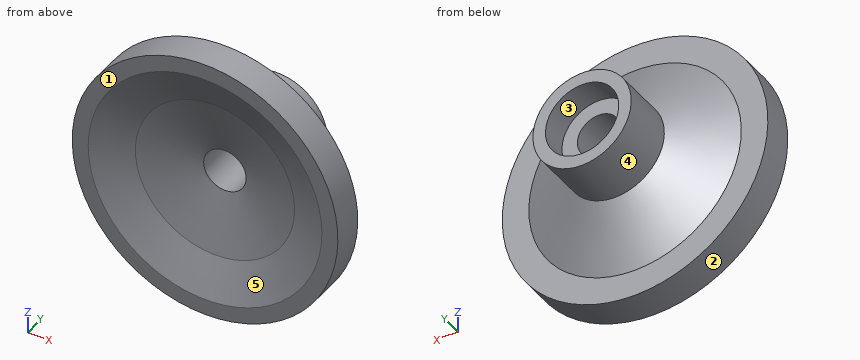
from build123d import *

# Parameters (mm, degrees)
SKETCH5_R          = 22
SKETCH7_R          = 15
SKETCH10_R         = 4
CUT_EXTRUDE1_DEPTH = 20
SKETCH11_R         = 6.9
CUT_EXTRUDE2_DEPTH = 5


with BuildPart() as part:
    # Sketch4 → Revolve1 (revolve)
    with BuildSketch(Plane.XY, mode=Mode.PRIVATE) as revolve1_sk:
        Polygon((25, 0), (25, 6), (20, 6), (9.25, 12), (9.25, 22), (0, 22), (0, 0), align=None)
    revolve(revolve1_sk.sketch.rotate(Axis((0, 0, 0), (0, 1, 0)), 90), axis=Axis((0, 0, 0), (0, 1, 0)))

    # Sketch5 → Cut-Loft1 section 0
    with BuildSketch(Plane.XZ):
        Circle(SKETCH5_R)
    # Sketch7 → Cut-Loft1 section 1
    with BuildSketch(Plane(origin=(0, 3, 0), x_dir=(-1, 0, 0), z_dir=(0, -1, 0))):
        Circle(SKETCH7_R)
    loft(mode=Mode.SUBTRACT)

    # Cut-Loft2: read off the stored shape, not the designer's step
    # Cut-Loft2: loft between two sections, ruled curve by curve
    cut_loft2_from = [
        Edge.make_bspline([(-3.999744183, 6, 0.04523797), (-4.090220122, 6, -7.954250395), (3.909268243, 6, -8.044726335), (3.999744183, 6, -0.04523797), (4.090220122, 6, 7.954250395), (-3.909268243, 6, 8.044726335), (-3.999744183, 6, 0.04523797)], [0, 0, 0, 0, 0.5, 0.5, 0.5, 1, 1, 1, 1], 3, [1, 0.333333333, 0.333333333, 1, 0.333333333, 0.333333333, 1]),
    ]
    cut_loft2_to = [
        Edge.make_bspline([(-14.242368289, 3, 4.706904028), (-23.656176345, 3, -23.777832549), (4.828560232, 3, -33.191640605), (14.242368289, 3, -4.706904028), (23.656176345, 3, 23.777832549), (-4.828560232, 3, 33.191640605), (-14.242368289, 3, 4.706904028)], [0, 0, 0, 0, 0.5, 0.5, 0.5, 1, 1, 1, 1], 3, [1, 0.333333333, 0.333333333, 1, 0.333333333, 0.333333333, 1]),
    ]
    cut_loft2 = Solid(Shell([*[Face.make_surface_from_curves(cut_loft2_from[k], cut_loft2_to[k]) for k in range(1)], Face(Wire(cut_loft2_from)), Face(Wire(cut_loft2_to))]))
    add(cut_loft2, mode=Mode.SUBTRACT)

    # Sketch10 → Cut-Extrude1 (cut)
    with BuildSketch(Plane.XZ.offset(-6)):
        with Locations(Location((0, 0, 0), (0, 0, 179.352))):
            Circle(SKETCH10_R)
    extrude(amount=-CUT_EXTRUDE1_DEPTH, mode=Mode.SUBTRACT)

    # Sketch11 → Cut-Extrude2 (cut)
    with BuildSketch(Plane(origin=(0, 22, 0), x_dir=(1, 0, 0), z_dir=(0, 1, 0))):
        with Locations(Location((0, 0, 0), (0, 0, 270))):
            Circle(SKETCH11_R)
    extrude(amount=-CUT_EXTRUDE2_DEPTH, mode=Mode.SUBTRACT)


solid = part.part
Here's how the part is built. I have some questions about the finished solid (model axes, mm). Face numbers are marked on the shaded views. A direction names the side the tool comes from. Coordinates: 2 decimals unless noted, no trailing zeros. Write each loop counter-clockwise with the first axis right and the second up, starting at its lowest first coordinate (ties: lowest second). Pieces come first, ordered by that corner, then holes.
Item 1: On a 3-axis mill with a long thin cutter (end or side, diameter ignored), from which of +Z, -Z, +X, -X, +Y, -Y can I reach the whole of each face in a straight line? I mean the marked faces 4 and 5. Say none if no direction works.
Item 2: I want a section at B-B on y = 15. Write out the boundary of the cut face in (x, z).
Item 3: I want a section at A-A on y = 10. Write out the boundary of the cut face in (x, z).
Item 4: If I drill on line 1 (X direction, y = 20.55, z = 0); line 2 (X direction, y = 14.25, z = 0); line 3 (Y direction, x = -10.5, z = 22), over which ranges is the centre line in solid material (lowest first)?
Item 5: Will these pins go through, and if not, where does the flat tip stop? pin 1 (11 mm diameter, centred on x = 0.5, z = -0.5, fed in from +Y); pin 2 (10 mm diameter, centred on x = 7.5, z = 12.5, fed in from +Y); pin 3 (6 mm diameter, centred on x = 3.5, z = -6, fed in from -Y).
Item 6: If we mould it in two halves opening along X, with no side actions, what happens to the marked faces 1, 2 and 3? For each: +X half, -X half, draft (parallel to the pull), parting line (faces both ways), or undercut.
Findings below:
1. face 4: +Y
1. face 5: -Y
2. outline: circle Ø18.5 at (0, 0); hole circle Ø8 at (0, 0)
3. outline: circle Ø25.67 at (0, 0); hole circle Ø8 at (0, 0)
4. line 1: x = -9.25 to -6.9, 6.9 to 9.25
4. line 2: x = -9.25 to -4, 4 to 9.25
4. line 3: y = 0 to 6
5. pin 1: stops at y = 17
5. pin 2: stops at y = 11.82
5. pin 3: stops at y = 4.36
6. face 1: draft
6. face 2: parting line
6. face 3: undercut
